The listing builds one solid part. Answer for the finished solid, in the listing's coordinates (mm). Coordinates: 2 decimals unless noted, no trailing zeros. Order: outer loops, then holes, each group sorted by start corner. A loop starts at its lowest first (then second) coordinate and runs counter-clockwise, first axis right, second up. Notation, with made-up numbers: (69.5, 62) -> (103.5, 62) arc R21 ccw to (103.5, 78) -> close; hole circle Ø5 at (22, -34). An arc over 180 degrees is marked (long way). Answer in a Markdown table with one row per item.
```python
from build123d import *

# Parameters (mm, degrees)
F0_W     = 355.6
F0_H     = 355.6
F1_DEPTH = 6.35
F2_R     = 6.35
F3_DEPTH = 25.4
F5_R     = 6.35
F6_DEPTH = 25.4


with BuildPart() as f1:
    # F0 (on Top) → F1 (new body)
    with BuildSketch(Plane.XY):
        with Locations((177.8, 177.8)):
            Rectangle(F0_W, F0_H)
    extrude(amount=F1_DEPTH)

    # F2 (on face) → F3 (cut)
    with BuildSketch(Plane.XY.offset(6.35)):
        with Locations((25.4, 228.6)):
            Circle(F2_R)
        with Locations((177.8, 330.2)):
            Circle(F2_R)
        with Locations((330.2, 228.6)):
            Circle(F2_R)
        with Locations((25.4, 127)):
            Circle(F2_R)
        with Locations((177.8, 25.4)):
            Circle(F2_R)
        with Locations((330.2, 127)):
            Circle(F2_R)
    extrude(amount=-F3_DEPTH, mode=Mode.SUBTRACT)

    # F5 (on face) → F6 (cut)
    with BuildSketch(Plane.XY.offset(6.35)):
        with Locations((25.4, 330.2)):
            Circle(F5_R)
        with Locations((330.2, 330.2)):
            Circle(F5_R)
        with Locations((25.4, 25.4)):
            Circle(F5_R)
        with Locations((330.2, 25.4)):
            Circle(F5_R)
    extrude(amount=-F6_DEPTH, mode=Mode.SUBTRACT)


solid = f1.part
```
(1) Find the intervals of material crossed by line 1 along X through (y, z) = (330.2, 5); line 2 along Y through (x, z) = (177.8, 2.25); line 3 along Y through (x, z) = (25.4, 1.5), in increasing order. Write a range as from..to.
Check values:
| item | result |
|---|---|
| line 1 | 0..19.05, 31.75..171.45, 184.15..323.85, 336.55..355.6 |
| line 2 | 0..19.05, 31.75..323.85, 336.55..355.6 |
| line 3 | 0..19.05, 31.75..120.65, 133.35..222.25, 234.95..323.85, 336.55..355.6 |
(2) A cutting plane is placed at B-B, the plane y = 25.4. Determine the outline of the cut face in (x, z), then the cut area to 3 significant figures.
Check values:
| item | result |
|---|---|
| outline | (0, 0) -> (19.05, 0) -> (19.05, 6.35) -> (0, 6.35) -> close; (31.75, 0) -> (171.45, 0) -> (171.45, 6.35) -> (31.75, 6.35) -> close; (184.15, 0) -> (323.85, 0) -> (323.85, 6.35) -> (184.15, 6.35) -> close; (336.55, 0) -> (355.6, 0) -> (355.6, 6.35) -> (336.55, 6.35) -> close |
| area | 2,020 mm² |
(3) For a pull along X with two mould halves and no side action, classify faces 1 (the cylindrical face through (333.614, 132.354, 3.219)), 2 (the flat face through (175, 180, 0)) as released by +X, released by -X, zero draft, split by the parting line, or undercut.
Check values:
| item | result |
|---|---|
| face 1 | undercut |
| face 2 | zero draft |
(4) A cutting plane is placed at C-C, the plane x = 177.8. Determine the outline of the cut face in (y, z).
Check values:
| item | result |
|---|---|
| outline | (0, 0) -> (19.05, 0) -> (19.05, 6.35) -> (0, 6.35) -> close; (31.75, 0) -> (323.85, 0) -> (323.85, 6.35) -> (31.75, 6.35) -> close; (336.55, 0) -> (355.6, 0) -> (355.6, 6.35) -> (336.55, 6.35) -> close |
(5) A cutting plane is placed at A-A, the plane x = 330.2. Determine the outline of the cut face in (y, z), then the cut area to 3 significant figures.
Check values:
| item | result |
|---|---|
| outline | (0, 0) -> (19.05, 0) -> (19.05, 6.35) -> (0, 6.35) -> close; (31.75, 0) -> (120.65, 0) -> (120.65, 6.35) -> (31.75, 6.35) -> close; (133.35, 0) -> (222.25, 0) -> (222.25, 6.35) -> (133.35, 6.35) -> close; (234.95, 0) -> (323.85, 0) -> (323.85, 6.35) -> (234.95, 6.35) -> close; (336.55, 0) -> (355.6, 0) -> (355.6, 6.35) -> (336.55, 6.35) -> close |
| area | 1,940 mm² |
(6) A flat-ended cylindrical pin translates along its axis: pin 1 (7.5 mm diameter, centred on x = 177.8, y = 330.2, fed in from +Z). Find the tip coordinate at first contact, or state that the pin passes through.
Check values:
| item | result |
|---|---|
| pin 1 | through |
